Read the model definition and answer for the solid it produces. Units are mm, in the model's axes. Round coordinates to 2 decimals unless told otherwise and drop trailing zeros. Order: outer loops, then holes, each group sorted by start corner. A loop starts at its lowest first (then second) coordinate and runs counter-clockwise, first axis right, second up. Notation, with made-up numbers: (82.25, 8.5) - (110.25, 8.5) arc R25 cw to (110.25, 45.5) - close; hole circle Ø11 at (-10.75, -25.5). An arc over 180 degrees is marked (long way). Answer as a JSON object with one key per item and string values. Group by question number.
Q1. A cutting plane is placed at C-C on z = 4. Determine the outline of the cut face in (x, y), and give its area (3 significant figures).
Q2. A cutting plane is placed at B-B on y = 0.9. Count the separate pieces of the cut face and the enclosed holes in it, and give its area (3 significant figures).
Q3. Given pin 1 Ø1.5 at (x, y) = (-21, 3.5) entering from -Z; pin 2 Ø4.5 at (x, z) = (0.07, 9.89) entering from +Y; pin 3 Ø2 at (x, z) = (-9.71, 0.11) entering from -Y, each flat-ended and moving along its own axis, determine where each tip first touches the part or whether it passes through.
Q4. Consider line 1 (X direction, y = 1.85, z = 0); line 2 (Z direction, x = -33.5, y = 1.8); line 3 (Y direction, x = 4, z = -8). Determine where each line is inside the solid, lowest interval first.
Q5. A cutting plane is placed at A-A on x = -63.5. Determine the outline of the cut face in (y, z), and give its area (3 significant figures).
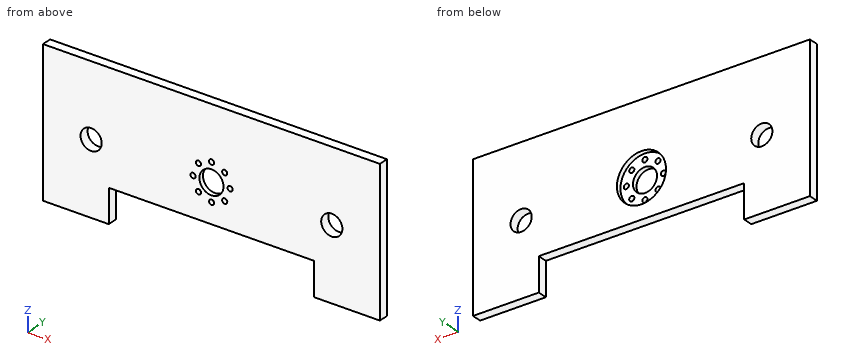
```python
from build123d import *

# Parameters (mm, degrees)
SKETCH1_W             = 177.8
SKETCH1_H             = 76.2
SKETCH1_R             = 5.588
BOSS_EXTRUDE1_DEPTH   = 5.08
SKETCH2_R             = 12.954
SKETCH2_R_2           = 0.712100007
CUT_EXTRUDE1_DEPTH    = 2.54
SKETCH4_R             = 6.35
CUT_EXTRUDE2_DEPTH    = 6.08
F_6_32_TAPPED_HOLE2_D = 2.7051
SKETCH9_W             = 108.359679772
SKETCH9_H             = 17.691365346
CUT_EXTRUDE7_DEPTH    = 5.08


with BuildPart() as part:
    # Sketch1 → Boss-Extrude1 (new body)
    with BuildSketch(Plane(origin=(0, 0, 0), x_dir=(1, 0, 0), z_dir=(0, 1, 0))):
        Rectangle(SKETCH1_W, SKETCH1_H)
        with Locations((-63.5, 0)):
            Circle(SKETCH1_R, mode=Mode.SUBTRACT)
        with Locations((63.5, 0)):
            Circle(SKETCH1_R, mode=Mode.SUBTRACT)
    extrude(amount=BOSS_EXTRUDE1_DEPTH)

    # Sketch2 → Cut-Extrude1 (cut)
    with BuildSketch(Plane(origin=(0, 5.08, 0), x_dir=(1, 0, 0), z_dir=(0, 1, 0))):
        Circle(SKETCH2_R)
        with Locations((6.980537549, -7.023044726)):
            Circle(SKETCH2_R_2, mode=Mode.SUBTRACT)
        with Locations((9.844740335, -0.108247513)):
            Circle(SKETCH2_R_2, mode=Mode.SUBTRACT)
        with Locations((-6.849056878, -7.023044726)):
            Circle(SKETCH2_R_2, mode=Mode.SUBTRACT)
        with Locations((0.065740335, -9.887247513)):
            Circle(SKETCH2_R_2, mode=Mode.SUBTRACT)
        with Locations((6.980537549, 6.8065497)):
            Circle(SKETCH2_R_2, mode=Mode.SUBTRACT)
        with Locations((0.065740335, 9.670752487)):
            Circle(SKETCH2_R_2, mode=Mode.SUBTRACT)
        with Locations((-6.849056878, 6.8065497)):
            Circle(SKETCH2_R_2, mode=Mode.SUBTRACT)
        with Locations((-9.713259665, -0.108247513)):
            Circle(SKETCH2_R_2, mode=Mode.SUBTRACT)
    extrude(amount=-CUT_EXTRUDE1_DEPTH, mode=Mode.SUBTRACT)

    # Sketch4 → Cut-Extrude2 (cut, through all)
    with BuildSketch(Plane(origin=(0, 5.08, 0), x_dir=(1, 0, 0), z_dir=(0, 1, 0))):
        Circle(SKETCH4_R)
    extrude(amount=-CUT_EXTRUDE2_DEPTH, mode=Mode.SUBTRACT)

    # #6-32 Tapped Hole2 (through all)
    with Locations(Plane(origin=(0, 2.54, 0), x_dir=(1, 0, 0), z_dir=(0, 1, 0))):
        with Locations((6.980537549, 6.8065497), (9.844740335, -0.108247513), (6.980537549, -7.023044726), (0.065740335, 9.670752487), (-6.849056878, 6.8065497), (-9.713259665, -0.108247513), (-6.849056878, -7.023044726), (0.065740335, -9.887247513)):
            Hole(F_6_32_TAPPED_HOLE2_D / 2)

    # Sketch9 → Cut-Extrude7 (cut)
    with BuildSketch(Plane(origin=(0, 0, 0), x_dir=(1, 0, 0), z_dir=(0, 1, 0))):
        with Locations((0, 29.254317327)):
            Rectangle(SKETCH9_W, SKETCH9_H)
    extrude(amount=CUT_EXTRUDE7_DEPTH, mode=Mode.SUBTRACT)


solid = part.part
```
Result set:
{
 "1": {"outline": "(-88.9, 0) - (-67.4, 0) - (-67.4, 5.08) - (-88.9, 5.08) - close; (-59.6, 0) - (-4.93, 0) - (-4.93, 2.54) - (-12.32, 2.54) - (-12.32, 5.08) - (-59.6, 5.08) - close; (4.93, 0) - (59.6, 0) - (59.6, 5.08) - (12.32, 5.08) - (12.32, 2.54) - (4.93, 2.54) - close; (67.4, 0) - (88.9, 0) - (88.9, 5.08) - (67.4, 5.08) - close", "area": "736 mm²"},
 "2": {"separate pieces": "1", "enclosed holes": "11", "area": "11,300 mm²"},
 "3": {"pin 1": "stops at z = -20.41", "pin 2": "stops at y = 2.54", "pin 3": "passes through"},
 "4": {"line 1": "x = -88.9 to -69.09, -57.91 to -11.06, -8.37 to -6.35, 6.35 to 8.5, 11.19 to 57.91, 69.09 to 88.9", "line 2": "z = -20.41 to 38.1", "line 3": "y = 0 to 2.54"},
 "5": {"outline": "(0, -38.1) - (5.08, -38.1) - (5.08, -5.59) - (0, -5.59) - close; (0, 5.59) - (5.08, 5.59) - (5.08, 38.1) - (0, 38.1) - close", "area": "330 mm²"}
}
